Could you check a few things on this model? Use its own coordinates, in mm. A direction names the side the tool comes from. Coordinates: 2 decimals unless noted, no trailing zeros. Order: outer loops, then holes, each group sorted by start corner. A loop starts at its lowest first (then second) coordinate and runs counter-clockwise, first axis right, second up.
Autodesk Inventor part; units mm, degrees
ref_plane "YZ Plane" through (0, 0, 0) normal (1, 0, 0) x (0, 1, 0)
ref_plane "XZ Plane" through (0, 0, 0) normal (0, 1, 0) x (-1, 0, 0)
ref_plane "XY Plane" through (0, 0, 0) normal (0, 0, 1) x (1, 0, 0)
sketch "Sketch1" plane through (0, 0, 0) normal (0, 1, 0) x (-1, 0, 0)
  line L0 (-145, -145) -> (145, -145)
  line L1 (145, -145) -> (145, 145)
  line L2 (145, 145) -> (-145, 145)
  line L3 (-145, 145) -> (-145, -145)
  line L4 (-145, -145) -> (145, 145) construction
  line L5 (145, -145) -> (-145, 145) construction
  circle A0 centre (0, 0) radius 60
  line L6 (135, 135) -> (135, -135) construction
  line L7 (135, -135) -> (-135, -135) construction
  line L8 (-135, -135) -> (-135, 135) construction
  line L9 (-135, 135) -> (135, 135) construction
  line L10 (145, 135) -> (125, 135) construction
  line L11 (125, 135) -> (125, -135) construction
  line L12 (-145, 135) -> (-125, 135) construction
  line L13 (-125, 135) -> (-125, -135) construction
  line L14 (-125, 135) -> (125, 135) construction
  line L15 (-125, -135) -> (125, -135) construction
  line L16 (135, 125) -> (135, -125) construction
  line L17 (-135, 125) -> (-135, -125) construction
  circle A1 centre (0, -135) radius 2.75
  line L18 (0, -135) -> (75, -135)
  line L19 (0, -135) -> (-75, -135)
  circle A2 centre (75, -135) radius 2.75
  circle A3 centre (-75, -135) radius 2.75
  line L20 (0, 135) -> (75, 135)
  line L21 (0, 135) -> (-75, 135)
  circle A4 centre (75, 135) radius 2.75
  circle A5 centre (0, 135) radius 2.75
  circle A6 centre (-75, 135) radius 2.75
  line L22 (135, 0) -> (135, -75)
  line L23 (135, 0) -> (135, 75)
  circle A7 centre (135, -75) radius 2.75
  circle A8 centre (135, 0) radius 2.75
  circle A9 centre (135, 75) radius 2.75
  line L24 (-135, 0) -> (-135, -75)
  line L25 (-135, 0) -> (-135, 75)
  circle A10 centre (-135, -75) radius 2.75
  circle A11 centre (-135, 0) radius 2.75
  circle A12 centre (-135, 75) radius 2.75
  dimension "d0" = 290
  dimension "d1" = 290
  dimension "d2" = 120
  dimension "d3" = 10
  dimension "d4" = 20
  dimension "d5" = 20
  dimension "d29" = 5.5
  dimension "d30" = 75
  dimension "d31" = 75
  dimension "d32" = 5.5
  dimension "d33" = 5.5
  dimension "d34" = 75
  dimension "d35" = 75
  dimension "d36" = 5.5
  dimension "d37" = 5.5
  dimension "d38" = 5.5
  dimension "d39" = 75
  dimension "d40" = 75
  dimension "d41" = 5.5
  dimension "d42" = 5.5
  dimension "d43" = 5.5
  dimension "d44" = 75
  dimension "d45" = 75
  dimension "d46" = 5.5
  dimension "d47" = 5.5
  dimension "d48" = 5.5
extrude "Extrusion1" add sketch "Sketch1" against normal blind 6 contours L3 L2 L1 L0 | L18 L19 A1 | A3 | A1 L19 L18 | A2 | L21 A5 L20 | L20 A5 L21 | A4 | A6 | L23 A8 L22 | L22 A8 L23 | A7 | A9 | L25 A11 L24 | L24 A11 L25 | A10 | A12
fillet "Fillet1" radius 8 4 edges at (-145, -3, -145) (-145, -3, 145) (145, -3, 145) (145, -3, -145)
extrude "Extrusion2" cut sketch "Sketch1" against normal through all contours L18 L19 A1 | A3 | A1 L19 L18 | A2 | L21 A5 L20 | L20 A5 L21 | A4 | A6 | L23 A8 L22 | L22 A8 L23 | A7 | A9 | L25 A11 L24 | L24 A11 L25 | A10 | A12
sketch "Sketch3" plane through (0, 0, 0) normal (0, 1, 0) x (1, 0, 0)
  line L0 (-71.5, 71.5) -> (71.5, 71.5)
  line L1 (71.5, 71.5) -> (71.5, -71.5)
  line L2 (71.5, -71.5) -> (-71.5, -71.5)
  line L3 (-71.5, -71.5) -> (-71.5, 71.5)
  line L4 (-71.5, 71.5) -> (71.5, -71.5) construction
  line L5 (71.5, 71.5) -> (-71.5, -71.5) construction
  point P0 (0, 0)
  dimension "d51" = 143
  dimension "d52" = 143
hole "Hole2" at (-71.5, 0, 71.5) at (-71.5, 0, -71.5) at (71.5, 0, -71.5) at (71.5, 0, 71.5) direction (0, -1, 0) diameter 5.5 end through all
sketch "Sketch4" plane through (0, 0, 0) normal (0, 1, 0) x (1, 0, 0)
  line L0 (0, 0) -> (-110, 0) construction
  line L1 (-145, 137) -> (-145, -137)
  arc A0 (-77.7817, 77.7817) -> (-77.7817, -77.7817) centre (0, 0) ccw
  arc A1 (-86.9199, 86.9199) -> (-86.9199, -86.9199) centre (0, 0) ccw
  line L2 (-77.7817, 77.7817) -> (-86.9199, 86.9199)
  line L3 (0, 0) -> (222.1817, 0) construction
  line L4 (-77.7817, -77.7817) -> (-86.9199, -86.9199)
  line L5 (0, 0) -> (151.3127, 0) construction
  dimension "d60" = 110
  dimension "d61" = 135
  dimension "d62" = 135
extrude "Extrusion3" cut sketch "Sketch4" against normal blind 10
fillet "Fillet2" radius 2 4 edges at (-77.7817, -3, -77.7817) (-86.9199, -3, -86.9199) (-86.9199, -3, 86.9199) (-77.7817, -3, 77.7817)
equation "\"d32\" = d29"
equation "\"d33\" = d29"
properties part number "BaseTopPlate" material "Aluminum"
Item 1: I need wall thicknesses on line 1 (Z direction, x = 135, y = -4); line 2 (Z direction, x = -71, y = -4.8). Which ranges of each line are inside material? Lowest first, please.
Item 2: Suppose I cut it at B-B (y = -4.9). Count the separate pieces of the cut face and the enclosed holes in it, and give its area (3 significant figures).
Item 3: Suppose I cut it at C-C (z = -48). List the corners of the cut face in (x, y) for me.
Item 4: For pin 1 Ø9 at (x, z) = (-135, 75) entering from -Y, with a flat end and sliding along its axis, tell me the tip position at first contact or that it passes through.
Item 5: Suppose I cut it at A-A (x = 48). List the corners of the cut face in (y, z) for me.
Item 6: Suppose I cut it at D-D (z = -14). List the corners of the cut face in (x, y) for me.
Item 7: Which directions (+Z, -Z, +X, -X, +Y, -Y) give clear straight access to the entire face, cutting with the end or side of a thin tool? Please do faces 1 (the face through (-142.719, -3.042, -142.594)), 2 (the face through (-122.916, -2.958, -1.323)).
Geometry results:
1. line 1: z = -145 to -77.75, -72.25 to -2.75, 2.75 to 72.25, 77.75 to 145
1. line 2: z = -145 to -74.2, -68.8 to 68.8, 74.2 to 145
2. separate pieces: 1
2. enclosed holes: 18
2. area: 70,000 mm2
3. outline: (-145, -6) - (-113.16, -6) - (-113.16, 0) - (-145, 0) - close; (-98.97, -6) - (-36, -6) - (-36, 0) - (-98.97, 0) - close; (36, -6) - (145, -6) - (145, 0) - (36, 0) - close
4. pin 1: stops at y = -6
5. outline: (-6, -145) - (0, -145) - (0, -36) - (-6, -36) - close; (-6, 36) - (0, 36) - (0, 145) - (-6, 145) - close
6. outline: (-145, -6) - (-122.12, -6) - (-122.12, 0) - (-145, 0) - close; (-109.11, -6) - (-58.34, -6) - (-58.34, 0) - (-109.11, 0) - close; (58.34, -6) - (145, -6) - (145, 0) - (58.34, 0) - close
7. face 1: -Z, -X, +Y, -Y
7. face 2: +Y, -Y
